Geometry: final body of the model. Coordinates: model frame, mm. A direction names the side the tool comes from. Give positions to 0.01 mm unless a question says otherwise; leave off trailing zeros. Order: outer loops, then holes, each group sorted by start corner. A loop starts at its lowest first (then second) coordinate and runs counter-clockwise, first axis right, second up. Notation, with made-up numbers: (-5, -18) - (42, -18) arc R20 ccw to (42, -13) - close; hole circle Ø9 at (86, -31). An arc over 180 degrees is marked (long way). One line per item, written item: value.
```python
from build123d import *

# Parameters (mm, degrees)
SKETCH1_R           = 1.4224
BOSS_EXTRUDE1_DEPTH = 1.5875
CUT_EXTRUDE1_DEPTH  = 31.574112518


with BuildPart() as part:
    # Sketch1 → Boss-Extrude1 (new body)
    with BuildSketch(Plane.XY):
        with BuildLine():
            Line((-14.952058744, -2.948480848), (-16.984058744, -2.948480848))
            Line((-16.984058744, -2.948480848), (-16.984058744, -5.5245))
            Line((-16.984058744, -5.5245), (-20.871224203, -5.5245))
            ThreePointArc((-20.871224203, -5.5245), (21.59, 0), (-20.871224203, 5.5245))
            Line((-20.871224203, 5.5245), (-16.984058744, 5.5245))
            Line((-16.984058744, 5.5245), (-16.984058744, 2.948480848))
            Line((-16.984058744, 2.948480848), (-14.952058744, 2.948480848))
            ThreePointArc((-14.952058744, 2.948480848), (-13.968818521, 6.093415226), (-12.332576282, 8.9535))
            Line((-12.332576282, 8.9535), (-7.9248, 7.366))
            Line((-7.9248, 7.366), (-7.9248, 3.302))
            Line((-7.9248, 3.302), (-5.6007, 3.302))
            Line((-5.6007, 3.302), (-5.6007, 14.173558463))
            ThreePointArc((-5.6007, 14.173558463), (-4.895856129, 14.43219293), (-4.179129857, 14.6558))
            Line((-4.179129857, 14.6558), (4.179129857, 14.6558))
            Line((4.179129857, 14.6558), (11.43, 14.6558))
            Line((11.43, 14.6558), (11.43, -0.8128))
            Line((11.43, -0.8128), (12.9413, -0.8128))
            Line((12.9413, -0.8128), (12.9413, -4.064))
            Line((12.9413, -4.064), (8.4582, -4.064))
            Line((8.4582, -4.064), (8.4582, -8.9154))
            Line((8.4582, -8.9154), (1.2573, -8.9154))
            Line((1.2573, -8.9154), (1.2573, -7.3406))
            Line((1.2573, -7.3406), (-0.7747, -8.8265))
            Line((-0.7747, -8.8265), (-3.273729572, -11.3919))
            Line((-3.273729572, -11.3919), (-5.093162196, -9.619538602))
            Line((-5.093162196, -9.619538602), (-4.769706241, -9.287492148))
            Line((-4.769706241, -9.287492148), (-9.167166743, -5.0038))
            Line((-9.167166743, -5.0038), (-14.395123673, -5.0038))
            ThreePointArc((-14.395123673, -5.0038), (-14.709533071, -3.985879682), (-14.952058744, -2.948480848))
        make_face()
        with Locations((0, 18.415)):
            Circle(SKETCH1_R, mode=Mode.SUBTRACT)
        with Locations((0, -18.415)):
            Circle(SKETCH1_R, mode=Mode.SUBTRACT)
    extrude(amount=BOSS_EXTRUDE1_DEPTH)

    # Sketch2 → Cut-Extrude1 (cut, through all)
    with BuildSketch(Plane.XY.offset(1.5875)):
        Polygon((-14.395123673, -5.0038), (-16.984058744, -5.5245), (-16.984058744, 5.5245), (-14.203432675, 5.5245), align=None)
    extrude(amount=-CUT_EXTRUDE1_DEPTH, mode=Mode.SUBTRACT)


solid = part.part
```
1) Section C-C, the plane x = 6. Return loops of the section in (y, z).
Answers below:
outline: (-20.74, 0) - (-8.92, 0) - (-8.92, 1.59) - (-20.74, 1.59) - close; (14.66, 0) - (20.74, 0) - (20.74, 1.59) - (14.66, 1.59) - close
2) First-contact query: pin 1 (0.8 mm diameter, centred on x = -6.5, z = 0.5, fed in from -Y); pin 2 (0.8 mm diameter, centred on x = 12, z = 0.5, fed in from -Y); pin 3 (0.8 mm diameter, centred on x = 11.5, z = 0.5, fed in from +Y); pin 4 (2.5 mm diameter, centred on x = 0, y = -18.415, fed in from -Z). Flat tips, straight axial feed; report the tip coordinate or a pass-through.
Answers below:
pin 1: y = -20.71
pin 2: y = -18.21
pin 3: y = 18.52
pin 4: through
3) Section D-D, the plane z = 0.7. Return loops of the section in (x, y) (1 decimal), then the cut area to 3 significant figures.
Answers below:
outline: (-20.9, -5.5) arc R21.6 ccw (long way) to (-20.9, 5.5) - (-14.2, 5.5) arc R15.2 cw to (-12.3, 9) - (-7.9, 7.4) - (-7.9, 3.3) - (-5.6, 3.3) - (-5.6, 14.2) arc R15.2 cw to (-4.2, 14.7) - (11.4, 14.7) - (11.4, -0.8) - (12.9, -0.8) - (12.9, -4.1) - (8.5, -4.1) - (8.5, -8.9) - (1.3, -8.9) - (1.3, -7.3) - (-0.8, -8.8) - (-3.3, -11.4) - (-5.1, -9.6) - (-4.8, -9.3) - (-9.2, -5) - (-14.4, -5) - (-17, -5.5) - close; hole circle Ø2.8 at (0, -18.4); hole circle Ø2.8 at (0, 18.4)
area: 871 mm^2
4) Material intervals for line 1 along Y through (x, z) = (0, 0.45); line 2 along X through (y, z) = (-0.5, 1.2); line 3 along Y through (x, z) = (2, 1.55), sorted ascending.
Answers below:
line 1: -21.59 to -19.84, -16.99 to -8.26, 14.66 to 16.99, 19.84 to 21.59
line 2: 11.43 to 21.58
line 3: -21.5 to -8.92, 14.66 to 21.5
5) Section B-B, the plane y = 4.5. Return loops of the section in (x, z).
Answers below:
outline: (-7.92, 0) - (-5.6, 0) - (-5.6, 1.59) - (-7.92, 1.59) - close; (11.43, 0) - (21.12, 0) - (21.12, 1.59) - (11.43, 1.59) - close
6) Set-up query: faces 1 (the face through (-4.17, -10.52, 0.78)), 2 (the face through (-12, -5.004, 1)). Return all of +Z, -Z, +X, -X, +Y, -Y with unobstructed straight access to the full face (end or side cutting, diameter ignored); none if empty.
Answers below:
face 1: +Z, -Z
face 2: +Z, -Z, -X
7) Mould query, pull axis X, two halves, no side actions, for faces 3 (the face through (21.572, -0.871, 0.783)), 4 (the face through (-7.925, 5, 1)), 5 (the face through (9.5, -4.5, 0)), 6 (the face through (5, -8.915, 1)). Classes: released by +X, released by -X, zero draft, split by the parting line, or undercut.
Answers below:
face 3: split by the parting line
face 4: undercut
face 5: zero draft
face 6: undercut
8) Section A-A, the plane x = 0. Return loops of the section in (y, z).
Answers below:
outline: (-21.59, 0) - (-19.84, 0) - (-19.84, 1.59) - (-21.59, 1.59) - close; (-16.99, 0) - (-8.26, 0) - (-8.26, 1.59) - (-16.99, 1.59) - close; (14.66, 0) - (16.99, 0) - (16.99, 1.59) - (14.66, 1.59) - close; (19.84, 0) - (21.59, 0) - (21.59, 1.59) - (19.84, 1.59) - close
